The listing builds one solid part. Answer for the finished solid, in the listing's coordinates (mm). Face numbers are marked on the shaded views. A direction names the side the tool comes from. Coordinates: 2 decimals unless noted, no trailing zeros. Write each loop counter-clockwise with the first axis right and the second up, starting at its lowest first coordinate (ties: lowest second). Pieces come first, ordered by that corner, then holes. Notation, with made-up numbers: M 35,85 L 63,85 A33 ccw 63,120 Z; hole C -15.75,-20.5 d2. An arc over 180 degrees is marked long. Write item = value, one per line. Start each with the question number.
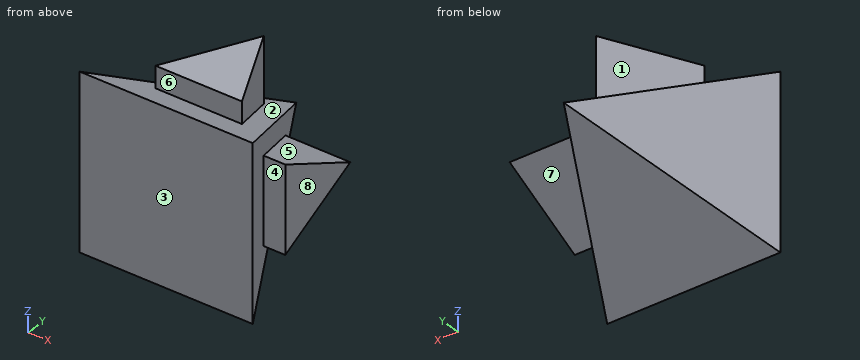
```python
from build123d import *

# Parameters (mm, degrees)
BOSS_EXTRUDE1_DEPTH   = 101.6
BODY_MOVE_COPY2_ANGLE = 90


with BuildPart() as part:
    # Sketch2 → Loft2 section 0
    with BuildSketch(Plane(origin=(0, 0, 0), x_dir=(1, 0, 0), z_dir=(0, 1, 0)), mode=Mode.PRIVATE) as loft2_s0:
        with BuildLine():
            Line((101.6, -101.6), (-101.6, -101.6))
            Line((-101.6, -101.6), (-101.6, 101.6))
            Line((-101.6, 101.6), (101.6, 101.6))
            Line((101.6, 101.6), (101.6, -101.6))
        make_face()
    loft([Vertex(0, 203.2, 0), loft2_s0.sketch])


with BuildPart() as body_2:
    # Sketch5 → Boss-Extrude1 (new body)
    with BuildSketch(Plane(origin=(0, 21.452394789, 0), x_dir=(1, 0, 0), z_dir=(0, 0, 1))):
        Polygon((0, 130.947605211), (-50.8, 29.347605211), (50.8, 29.347605211), align=None)
    extrude(amount=BOSS_EXTRUDE1_DEPTH)


with BuildPart() as body_3:
    # Body-Move/Copy2: copy of body 2
    add(body_2.part.rotate(Axis((0, 0, 0), (0, 1, 0)), BODY_MOVE_COPY2_ANGLE))


with BuildPart() as part_1:
    add(part.part)

    # Combine1: union body 2, body 3
    add(body_2.part)
    add(body_3.part)


solid = part_1.part
```
1. The part is cut by section B-B, the plane x = -36. Write down the section's boundary in (y, z).
2. For a pull along Y with two mould halves and no side action, classify the marked faces 1, 2, 3 and 4 as pulls with the +Y half, pulls with the -Y half, needs draft (parallel to the pull), parting line crosses it, or undercut.
3. The part is cut by section D-D, the plane z = -27.5. Write down the section's boundary in (x, y), and give its area (3 significant figures).
4. Straight lines are drawn through the part: L1, parallel to Y at x = 21, z = 83; L2, parallel to Z at x = -3, y = 54.5; L3, parallel to Y at x = -17, z = -91. For each, find the intervals that lie inside material, in ascending order. Write a range as [from, to].
5. The part is cut by section A-A, the plane z = 89. Write down the section's boundary in (x, y), and give its area (3 significant figures).
6. The part is cut by section C-C, the plane y = 69. Write down the section's boundary in (x, z), and give its area (3 significant figures).
7. For the marked faces 5, 6, 7 and 8, determine the directions among +Z, -Z, +X, -X, +Y, -Y from which every point of the face is accessible in a straight line to the end or side of a thin tool.
8. Each of these flat-tipped pins is pushed along its axis until it touches: pin 1 (6 mm diameter, centred on x = -80, z = -68, fed in from +Y); pin 2 (10 mm diameter, centred on x = -8.5, z = -74, fed in from +Y); pin 3 (1.5 mm diameter, centred on x = 23.5, y = 25.5, fed in from -Z) (3 decimals). Where does it stop, or does it pass through?
Solution:
q1.outline = M 0,-101.6 L 131.2,-36 L 131.2,36 L 80.4,61.4 L 80.4,101.6 L 50.8,101.6 L 50.8,76.2 L 0,101.6 Z
q2.face_1 = pulls with the +Y half
q2.face_2 = undercut
q2.face_3 = pulls with the -Y half
q2.face_4 = undercut
q3.outline = M -101.6,0 L 101.6,0 L 76.2,50.8 L 101.6,50.8 L 101.6,97.4 L 52.9,97.4 L 27.5,148.2 L -27.5,148.2 Z
q3.area = 20,900 mm^2
q4.L1 = [0, 37.2], [50.8, 110.4]
q4.L2 = [-74.35, 101.6]
q4.L3 = [0, 21.2]
q5.outline = M -101.6,0 L 101.6,0 L 89,25.2 L -89,25.2 Z; M -50.8,50.8 L 50.8,50.8 L 0,152.4 Z
q5.area = 9,960 mm^2
q6.outline = M -67.1,-67.1 L 67.1,-67.1 L 67.1,-41.7 L 101.6,-41.7 L 101.6,41.7 L 67.1,41.7 L 67.1,67.1 L 41.7,67.1 L 41.7,101.6 L -41.7,101.6 L -41.7,67.1 L -67.1,67.1 Z
q6.area = 23,800 mm^2
q7.face_5 = +Z, +X, +Y
q7.face_6 = +Z, +X, -X
q7.face_7 = -Z, +X, +Y
q7.face_8 = +Z, -Z, +X, +Y, -Y
q8.pin_1 = 49.2
q8.pin_2 = 65.2
q8.pin_3 = -89.225
